Geometry: final body of the model. Coordinates: model frame, mm. A direction names the side the tool comes from. Give positions to 0.01 mm unless a question says otherwise; leave off trailing zeros. Order: outer loops, then holes, each group sorted by start corner. A loop starts at its lowest first (then second) coordinate and runs counter-clockwise, first axis right, second up. Notation, with made-up numbers: M -24.75,-1.5 L 26.25,-1.5 A21 ccw 26.25,30.5 Z; hole C -7.5,-15.5 d1. An arc over 180 degrees is marked long. One line per item, written item: value. Start each with the question number.
```python
from build123d import *

# Parameters (mm, degrees)
ESQUISSE1_W                                        = 47
ESQUISSE1_H                                        = 39
BOSS_EXTRU_1_DEPTH                                 = 22
CHAMBRAGE_POUR_VIS_T_TE_RONDE_BOMB_E_M_D           = 3
CHAMBRAGE_POUR_VIS_T_TE_RONDE_BOMB_E_M_CBORE_D     = 5.8
CHAMBRAGE_POUR_VIS_T_TE_RONDE_BOMB_E_M_CBORE_DEPTH = 17
ENL_V_MAT_EXTRU_1_DEPTH                            = 14
CONG_1_R                                           = 5
CONG_2_R                                           = 2
ESQUISSE6_R                                        = 11.25
ESQUISSE6_R_2                                      = 9.25
ENL_V_MAT_EXTRU_2_DEPTH                            = 15
ESQUISSE8_R                                        = 2.5
ENL_V_MAT_EXTRU_3_DEPTH                            = 1
BOSS_EXTRU_5_DEPTH                                 = 1
R_P_TITION_CIRCULAIRE1_COUNT                       = 3
CONG_3_R                                           = 2
CONG_4_R                                           = 0.2


with BuildPart() as part:
    # Esquisse1 → Boss.-Extru.1 (new body)
    with BuildSketch(Plane(origin=(0, 0, 0), x_dir=(1, 0, 0), z_dir=(0, 1, 0))):
        Rectangle(ESQUISSE1_W, ESQUISSE1_H)
    extrude(amount=BOSS_EXTRU_1_DEPTH)

    # Chambrage pour vis à tête ronde bombée M31 (through all)
    with Locations(Plane(origin=(0, 22, 0), x_dir=(1, 0, 0), z_dir=(0, 1, 0))):
        with Locations((-19.5, -15), (19.5, 15)):
            CounterBoreHole(CHAMBRAGE_POUR_VIS_T_TE_RONDE_BOMB_E_M_D / 2, CHAMBRAGE_POUR_VIS_T_TE_RONDE_BOMB_E_M_CBORE_D / 2, CHAMBRAGE_POUR_VIS_T_TE_RONDE_BOMB_E_M_CBORE_DEPTH)

    # Esquisse5 → Enlèv. mat.-Extru.1 (cut)
    with BuildSketch(Plane(origin=(0, 22, 0), x_dir=(1, 0, 0), z_dir=(0, 1, 0))):
        with BuildLine():
            Line((-23.5, -8.1), (-23.5, -19.5))
            Line((-23.5, -19.5), (-12.1, -19.5))
            ThreePointArc((-12.1, -19.5), (-15.281980515, -18.181980515), (-16.6, -15))
            ThreePointArc((-16.6, -15), (-17.449390335, -12.949390335), (-19.5, -12.1))
            ThreePointArc((-19.5, -12.1), (-22.328427125, -10.928427125), (-23.5, -8.1))
        make_face()
        with BuildLine():
            Line((23.5, 8.1), (23.5, 19.5))
            Line((23.5, 19.5), (12.1, 19.5))
            ThreePointArc((12.1, 19.5), (15.281980515, 18.181980515), (16.6, 15))
            ThreePointArc((16.6, 15), (17.449390335, 12.949390335), (19.5, 12.1))
            ThreePointArc((19.5, 12.1), (22.328427125, 10.928427125), (23.5, 8.1))
        make_face()
    extrude(amount=-ENL_V_MAT_EXTRU_1_DEPTH, mode=Mode.SUBTRACT)

    # Congé1
    cong_1_edges = [part.edges().sort_by_distance(p)[0] for p in [
        (-23.5, 4, 19.5),
        (23.5, 4, -19.5),
        (23.5, 11, 19.5),
        (-23.5, 11, -19.5),
    ]]
    fillet(cong_1_edges, radius=CONG_1_R)

    # Congé2
    cong_2_edges = [part.edges().sort_by_distance(p)[0] for p in [
        (-17.449390335, 22, 12.949390335),
        (3.2, 22, 19.5),
        (-15.281980515, 22, 18.181980515),
        (-22.328427125, 22, 10.928427125),
        (17.449390335, 22, -12.949390335),
        (-3.2, 22, -19.5),
        (15.281980515, 22, -18.181980515),
        (22.328427125, 22, -10.928427125),
        (23.5, 22, 3.2),
        (-23.5, 22, -3.2),
        (-22.035533906, 22, -18.035533906),
        (22.035533906, 22, 18.035533906),
    ]]
    fillet(cong_2_edges, radius=CONG_2_R)

    # Esquisse6 → Enlèv. mat.-Extru.2 (cut)
    with BuildSketch(Plane(origin=(0, 22, 0), x_dir=(1, 0, 0), z_dir=(0, 1, 0))):
        with Locations(Location((-8.5, 4.5, 0), (0, 0, 270))):
            Circle(ESQUISSE6_R)
        with Locations(Location((-8.5, 4.5, 0), (0, 0, 270))):
            Circle(ESQUISSE6_R_2, mode=Mode.SUBTRACT)
    extrude(amount=-ENL_V_MAT_EXTRU_2_DEPTH, mode=Mode.SUBTRACT)

    # Esquisse8 → Enlèv. mat.-Extru.3 (cut)
    with BuildSketch(Plane(origin=(0, 22, 0), x_dir=(1, 0, 0), z_dir=(0, 1, 0))):
        with Locations(Location((-8.5, 4.5, 0), (0, 0, 270))):
            Circle(ESQUISSE8_R)
    extrude(amount=-ENL_V_MAT_EXTRU_3_DEPTH, mode=Mode.SUBTRACT)

    # Esquisse7 → Boss.-Extru.5 (add, symmetric)
    with BuildSketch(Plane.XY.offset(-4.5)):
        with BuildLine():
            Line((-20.21694009, 22), (-11, 22))
            Line((-11, 22), (-13.641435578, 22.66096111))
            ThreePointArc((-13.641435578, 22.66096111), (-14.200146525, 22.745896439), (-14.764873034, 22.724544554))
            Line((-14.764873034, 22.724544554), (-20.21694009, 22))
        make_face()
    boss_extru_5 = extrude(amount=BOSS_EXTRU_5_DEPTH, both=True)

    # Répétition circulaire1: Boss.-Extru.5 ×3 about axis
    r_p_tition_circulaire1_axis = Axis((-8.5, 0, -4.5), (0, 1, 0))
    for i in range(1, R_P_TITION_CIRCULAIRE1_COUNT):
        add(boss_extru_5.rotate(r_p_tition_circulaire1_axis, i * 360 / R_P_TITION_CIRCULAIRE1_COUNT))

    # Congé3
    cong_3_edges = [part.edges().sort_by_distance(p)[0] for p in [
        (-20.21694009, 22, -4.5),
        (-2.641529955, 22, 5.647167773),
        (-2.641529955, 22, -14.647167773),
    ]]
    fillet(cong_3_edges, radius=CONG_3_R)

    # Congé4
    cong_4_edges = [part.edges().sort_by_distance(p)[0] for p in [
        (-8.5, 21, -7),
    ]]
    fillet(cong_4_edges, radius=CONG_4_R)


solid = part.part
```
Q1. Section query A-A on y = 11.5. Return loops of the section in (x, z).
Q2. Ray query, line 1 along Z through (x, y) = (-8.5, 16.25); line 2 along X through (y, z) = (19, -4.5); line 3 along X through (y, z) = (19, -10). Return the intervals inside material, ascending. Write a range as [from, to].
Q3. Set-up query: faces 1 (the face through (-6.611, 22.326, -7.8)), 2 (the face through (-15.247, 14.084, 18.217)), 3 (the face through (-10.72, 21.61, -3.35)), 4 (the face through (-6.265, 22.297, -10.37)). Return all of +Z, -Z, +X, -X, +Y, -Y with unobstructed straight access to the full face (end or side cutting, diameter ignored); none if empty.
Q4. Contact query for flat-ended pins moving along their axis: pin 1 (9 mm diameter, centred on x = 17.5, z = -14, fed in from +Y); pin 2 (3 mm diameter, centred on x = 15.5, y = 13, fed in from -Z); pin 3 (2 mm diameter, centred on x = -3, z = 3.5, fed in from -Y); pin 4 (0.8 mm diameter, centred on x = -14.5, y = 22.5, fed in from -Z). Output: stop coordinate, or through.
Results below:
1. outline: M -23.5,-14.5 A5 ccw -18.5,-19.5 L 12.1,-19.5 A4.5 ccw 16.6,-15 A2.9 cw 19.5,-12.1 A4 ccw 23.5,-8.1 L 23.5,14.5 A5 ccw 18.5,19.5 L -12.1,19.5 A4.5 ccw -16.6,15 A2.9 cw -19.5,12.1 A4 ccw -23.5,8.1 Z; C -8.5,-4.5 d18.5; hole C -8.5,-4.5 d22.5
2. line 1: [-19.5, -15.75], [-13.75, 4.75], [6.75, 19.5]
2. line 2: [-23.5, -19.75], [-17.75, 0.75], [2.75, 23.5]
2. line 3: [-23.5, -18.31], [-15.94, -1.06], [1.31, 23.02]
3. face 1: -X, +Y
3. face 2: +Z, -X, +Y
3. face 3: +Y
3. face 4: -Z, -X, +Y
4. pin 1: y = 22
4. pin 2: z = -19.08
4. pin 3: y = 0
4. pin 4: z = -5.5
